For this review, use the dimensioned drawing (mm, ordinates from the lowest corner) and the shaded views. Give positions to 0.01 mm unless a question says otherwise; leave off trailing zeros. Write each loop counter-clockwise with the first axis right and the second up, starting at its lowest first coordinate (ties: lowest second). Pieces come first, ordered by that corner, then holes.
1) We need section A-A on x = 62. Give the boundary of the cut face in (y, z).
2) We need section B-B on z = 60.5. Give the boundary of the cut face in (x, y).
3) Wall thickness on line 1 along X through (y, z) = (0.55, 59); line 2 along X through (y, z) = (1.1, 39); line 3 along X through (y, z) = (1.8, 4.5) (1 decimal): over which ranges is each line inside the solid? List them lowest first.
4) We need section D-D on x = 43. Give the boundary of the cut face in (y, z).
5) We need section C-C on y = 0.45. Give the number of separate pieces and of enclosed holes in the cut face, and give its area (3 significant figures).
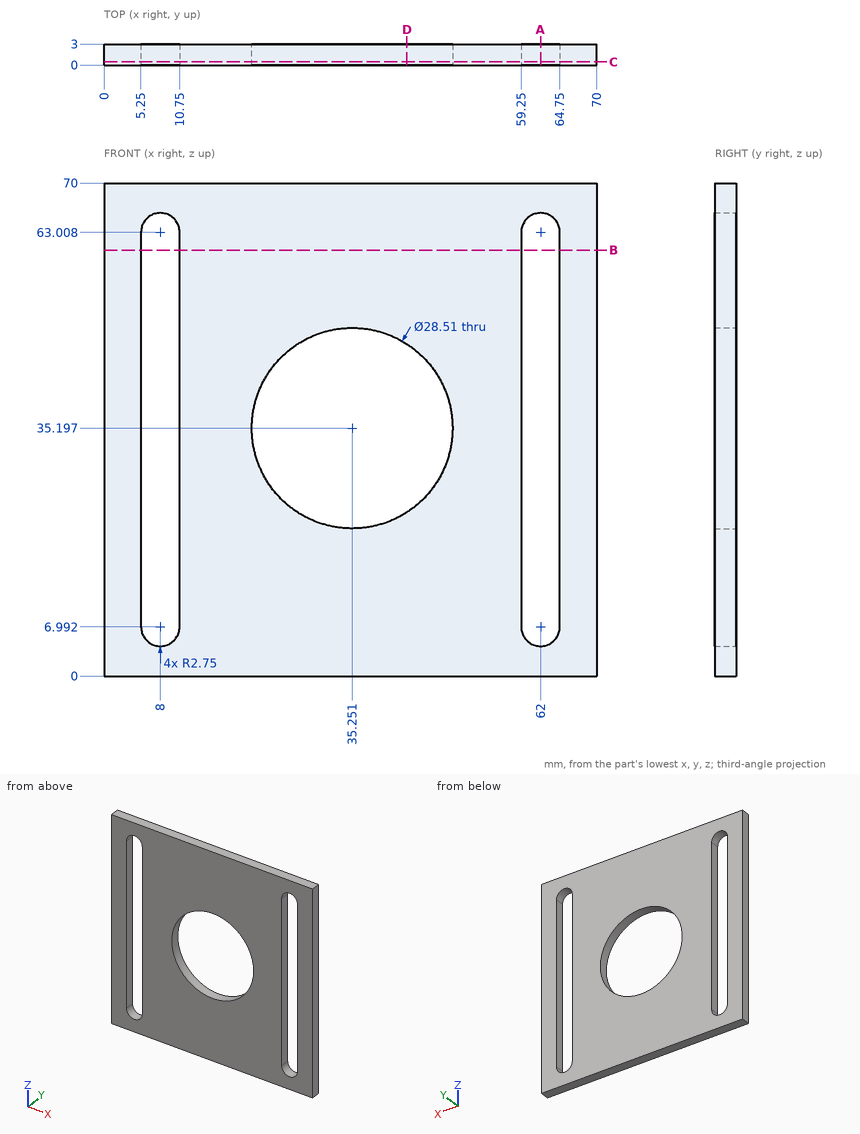
Results list:
1. outline: (0, 0) - (3, 0) - (3, 4.24) - (0, 4.24) - close; (0, 65.76) - (3, 65.76) - (3, 70) - (0, 70) - close
2. outline: (0, 0) - (5.25, 0) - (5.25, 3) - (0, 3) - close; (10.75, 0) - (59.25, 0) - (59.25, 3) - (10.75, 3) - close; (64.75, 0) - (70, 0) - (70, 3) - (64.75, 3) - close
3. line 1: x = 0 to 5.25, 10.75 to 59.25, 64.75 to 70
3. line 2: x = 0 to 5.25, 10.75 to 21.51, 48.99 to 59.25, 64.75 to 70
3. line 3: x = 0 to 6.8, 9.2 to 60.8, 63.2 to 70
4. outline: (0, 0) - (3, 0) - (3, 23.23) - (0, 23.23) - close; (0, 47.16) - (3, 47.16) - (3, 70) - (0, 70) - close
5. separate pieces: 1
5. enclosed holes: 3
5. area: 3,600 mm2
